Work out the finished part from the listing and answer in its coordinate system (mm). Face numbers are marked on the shaded views. A direction names the side the tool comes from. Coordinates: 2 decimals unless noted, no trailing zeros. Order: outer loops, then holes, each group sorted by start corner. A loop starts at its lowest first (then second) coordinate and runs counter-clockwise, first axis right, second up. Notation, with made-up numbers: (-10, 84) - (-2, 84) arc R11 cw to (-2, 97) - close; hole circle Ø1 at (55.25, 77.5). An arc over 180 degrees is marked (long way). Answer as a JSON object with one key per item and string values. Group by question number.
1) Section A-A (x = 12) is taken. Give the vertices of the cut face in (y, z), plus the area to 3 significant figures.
2) The mould has two halves that part along Y. Classify the marked faces 1, 2, 3 and 4: released by +Y, released by -Y, zero draft, split by the parting line, or undercut.
3) Each of these flat-tipped pins is pushed along its axis until it touches: P1, Ø8, axis at x = 3.5, y = 2, coming from the -Z side; P2, Ø8, axis at x = -4, z = 0, coming from the +Y side; P3, Ø1.5, axis at x = 3, z = -1.5, coming from the -Y side; P4, Ø10, axis at y = -3.5, z = -1, coming from the -X side. Where does it stop, or does it pass through?
4) A tool of negligible diameter and unlimited length cuts with its end or side. For the marked faces 5, 6 and 7, from which of +Z, -Z, +X, -X, +Y, -Y can it reach the whole face along a straight path? Write none if from no direction.
5) Find the intervals of material crossed by line 1 along Y through (x, z) = (7.25, 0); line 2 along Y through (x, z) = (10.5, 0); line 3 along Z through (x, y) = (-12.5, -0.5), in increasing order.
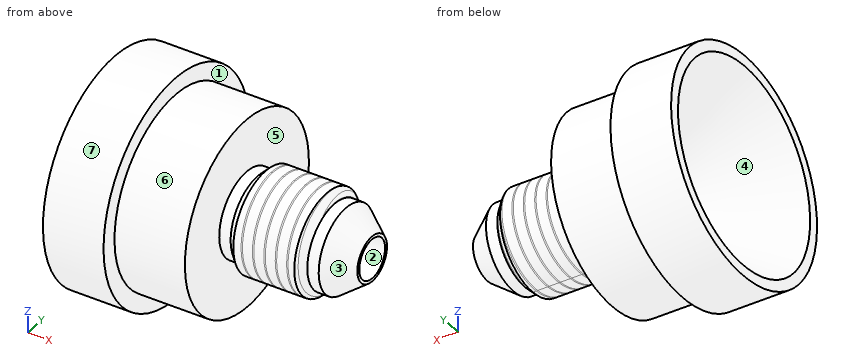
from build123d import *

# Parameters (mm, degrees)
CUT_SWEEP1_PITCH = 1.27


with BuildPart() as part:
    # Sketch1 → Revolve1 (revolve)
    with BuildSketch(Plane.XY, mode=Mode.PRIVATE) as revolve1_sk:
        Polygon((-14.2875, 12.3444), (-14.2875, 11.176), (-2.355243782, 2.1844), (14.2875, 2.1844), (14.2875, 2.51206), (14.2875, 5.55625), (10.247723424, 5.55625), (0.3175, 5.55625), (0.3175, 10.4902), (-7.5311, 10.4902), (-7.5311, 12.3444), align=None)
    revolve(revolve1_sk.sketch.rotate(Axis((-14.2875, 0, 0), (1, 0, 0)), 90), axis=Axis((-14.2875, 0, 0), (1, 0, 0)))

    # Cut-Sweep1: the profile of Sketch4 profile screwed along a right-hand helix of 11 turns, 8 arcs to a turn; built about Z, then put on its axis
    cut_sweep1_z = Axis((0, 0, 0), (0, 0, 1))
    cut_sweep1_corners = [(5.55655, 0, 0.000173205), (5.55655, 0, -1.111423205), (4.731360803, 0, -0.635), (4.731360803, 0, -0.47625)]
    with BuildLine(mode=Mode.PRIVATE) as cut_sweep1_profile:
        Line(cut_sweep1_corners[0], cut_sweep1_corners[1])
        Line(cut_sweep1_corners[1], cut_sweep1_corners[2])
        Line(cut_sweep1_corners[2], cut_sweep1_corners[3])
        Line(cut_sweep1_corners[3], cut_sweep1_corners[0])
    cut_sweep1_cap = Face(cut_sweep1_profile.wire())
    cut_sweep1_turn_angles = [0, 22.5, 45, 67.5, 90, 112.5, 135, 157.5, 180, 202.5, 225, 247.5, 270, 292.5, 315, 337.5, 360]
    cut_sweep1_turn_weights = [1, 0.9238795325112867, 1, 0.9238795325112867, 1, 0.9238795325112867, 1, 0.9238795325112867, 1, 0.9238795325112867, 1, 0.9238795325112867, 1, 0.9238795325112867, 1, 0.9238795325112867, 1]
    cut_sweep1_turn_rails = [Edge.make_bspline([Vector(p[0], p[1], 0).rotate(cut_sweep1_z, cut_sweep1_turn_angles[k]) / cut_sweep1_turn_weights[k] + Vector(0, 0, p[2] + CUT_SWEEP1_PITCH * cut_sweep1_turn_angles[k] / 360) for k in range(17)], [0, 0, 0, 1, 1, 2, 2, 3, 3, 4, 4, 5, 5, 6, 6, 7, 7, 8, 8, 8], 2, cut_sweep1_turn_weights) for p in cut_sweep1_corners]
    cut_sweep1_turn_sides = [Face.make_surface_from_curves(cut_sweep1_turn_rails[p[0]], cut_sweep1_turn_rails[p[1]]) for p in [(0, 1), (1, 2), (2, 3), (3, 0)]]
    cut_sweep1_turn = Solid(Shell([*cut_sweep1_turn_sides, cut_sweep1_cap, cut_sweep1_cap.rotate(cut_sweep1_z, 360).moved(Location((0, 0, CUT_SWEEP1_PITCH * 360 / 360)))]))
    cut_sweep1_each = [*[cut_sweep1_turn.moved(Location((0, 0, CUT_SWEEP1_PITCH * i))) for i in range(11)]]
    add(Plane(origin=(14.2875, 0, 0), x_dir=(0, 1, 0), z_dir=(-1, 0, 0)) * Compound([cut_sweep1_each[i] for i in range(0, 11, 2)]), mode=Mode.SUBTRACT)
    add(Plane(origin=(14.2875, 0, 0), x_dir=(0, 1, 0), z_dir=(-1, 0, 0)) * Compound([cut_sweep1_each[i] for i in range(1, 11, 2)]), mode=Mode.SUBTRACT)

    # Sketch5 → Cut-Revolve1 (revolve, cut)
    with BuildSketch(Plane.XY, mode=Mode.PRIVATE) as cut_revolve1_sk:
        Polygon((14.2875, 2.51206), (11.409802239, 4.680560803), (10.139802239, 4.680560803), (9.264113042, 5.55625), (14.2875, 5.55625), align=None)
        Polygon((0.3175, 5.55625), (0.3175, 4.680560803), (1.5875, 4.680560803), (2.463189197, 5.55625), align=None)
    revolve(cut_revolve1_sk.sketch.rotate(Axis((0, 0, 0), (-1, 0, 0)), 90), axis=Axis((0, 0, 0), (-1, 0, 0)), mode=Mode.SUBTRACT)

    # Sketch6 → Revolve2 (revolve)
    with BuildSketch(Plane.XY, mode=Mode.PRIVATE) as revolve2_sk:
        Polygon((2.463189197, 5.55625), (1.5875, 4.680560803), (10.139802239, 4.680560803), (9.264113042, 5.55625), align=None)
    revolve(revolve2_sk.sketch.rotate(Axis((0, 0, 0), (1, 0, 0)), 270), axis=Axis((0, 0, 0), (1, 0, 0)))


solid = part.part
Report:
{
 "1": {"outline": "circle Ø8.47 at (0, 0); hole circle Ø4.37 at (0, 0)", "area": "41.4 mm²"},
 "2": {"face 1": "zero draft", "face 2": "undercut", "face 3": "split by the parting line", "face 4": "undercut"},
 "3": {"P1": "stops at z = -10.49", "P2": "stops at y = 12.34", "P3": "stops at y = -5.51", "P4": "stops at x = -10.92"},
 "4": {"face 5": "none", "face 6": "+X", "face 7": "+X, -X"},
 "5": {"line 1": "y = -5.56 to -2.18, 2.18 to 5.56", "line 2": "y = -4.68 to -2.18, 2.18 to 4.68", "line 3": "z = -12.33 to -9.82, 9.82 to 12.33"}
}
